The model under review builds one solid part; all positions refer to its coordinate system, in mm. Face numbers are marked on the shaded views. A direction names the side the tool comes from. Coordinates: 2 decimals unless noted, no trailing zeros. Loops run counter-clockwise (first coordinate to the right, second up) from the corner with the lowest first, then second, coordinate; pieces in that order, holes last. Notation, with made-up numbers: M 33.5,8.25 L 76.5,8.25 A24 ccw 76.5,38.25 Z; hole C 46,1.25 d6. An arc over 180 degrees is marked long. Return JSON: item names as keys, results as strings.
```python
from build123d import *

# Parameters (mm, degrees)
SKETCH1_R               = 9.35355
BOSS_EXTRUDE1_DEPTH     = 2.38125
BOSS_EXTRUDE2_START     = 6.35
SKETCH2_R               = 9.35355
SKETCH2_W               = 3.429
SKETCH2_H               = 3.429
BOSS_EXTRUDE2_DEPTH     = 6.35
SKETCH3_W               = 3.429
SKETCH3_H               = 3.429
SKETCH3_R               = 1.25
BOSS_EXTRUDE3_DEPTH     = 1
CUT_EXTRUDE1_DEPTH      = 20.29812849
CUT_EXTRUDE1_DEPTH_BACK = 20.29812849
SKETCH4_OUTSIDE_W       = 26.28
SKETCH4_OUTSIDE_H       = 26.279
SKETCH4_OUTSIDE_R       = 7.14375


with BuildPart() as part:
    # Sketch1 → Boss-Extrude1 (new body)
    with BuildSketch(Plane.XY.offset(20.11015)):
        with Locations((0, 5.0927)):
            Circle(SKETCH1_R)
        with BuildLine():
            Line((-2.032, 2.088352317), (-2.032, -1.4351))
            ThreePointArc((-2.032, -1.4351), (0, -3.4671), (2.032, -1.4351))
            Line((2.032, -1.4351), (2.032, 2.088352317))
            ThreePointArc((2.032, 2.088352317), (3.627, 5.0927), (2.032, 8.097047683))
            Line((2.032, 8.097047683), (2.032, 11.6205))
            ThreePointArc((2.032, 11.6205), (0, 13.6525), (-2.032, 11.6205))
            Line((-2.032, 11.6205), (-2.032, 8.097047683))
            ThreePointArc((-2.032, 8.097047683), (-3.627, 5.0927), (-2.032, 2.088352317))
        make_face(mode=Mode.SUBTRACT)
    extrude(amount=-BOSS_EXTRUDE1_DEPTH)

    # Sketch2 → Boss-Extrude2 (add)
    with BuildSketch(Plane.XY.offset(20.11015).offset(BOSS_EXTRUDE2_START)):
        with Locations((0, 5.0927)):
            Circle(SKETCH2_R)
        with Locations((0, 5.0927)):
            Rectangle(SKETCH2_W, SKETCH2_H, mode=Mode.SUBTRACT)
    extrude(amount=-BOSS_EXTRUDE2_DEPTH)

    # Sketch3 → Boss-Extrude3 (add)
    with BuildSketch(Plane(origin=(0, 0, 20.11015), x_dir=(-1, 0, 0), z_dir=(0, 0, -1))):
        with Locations((0, 5.0927)):
            Rectangle(SKETCH3_W, SKETCH3_H)
        with Locations((0, 5.0927)):
            Circle(SKETCH3_R, mode=Mode.SUBTRACT)
    extrude(amount=-BOSS_EXTRUDE3_DEPTH)

    # Sketch4 outside → Cut-Extrude1 (cut, two sides: drawn at the far end of the back side and taken through both)
    with BuildSketch(Plane(origin=(0, 0, 17.7289), x_dir=(-1, 0, 0), z_dir=(0, 0, -1)).offset(-CUT_EXTRUDE1_DEPTH_BACK)):
        with Locations((0, 5.0925)):
            Rectangle(SKETCH4_OUTSIDE_W, SKETCH4_OUTSIDE_H)
        with Locations((0, 5.0927)):
            Circle(SKETCH4_OUTSIDE_R, mode=Mode.SUBTRACT)
    extrude(amount=CUT_EXTRUDE1_DEPTH + CUT_EXTRUDE1_DEPTH_BACK, mode=Mode.SUBTRACT)


solid = part.part
```
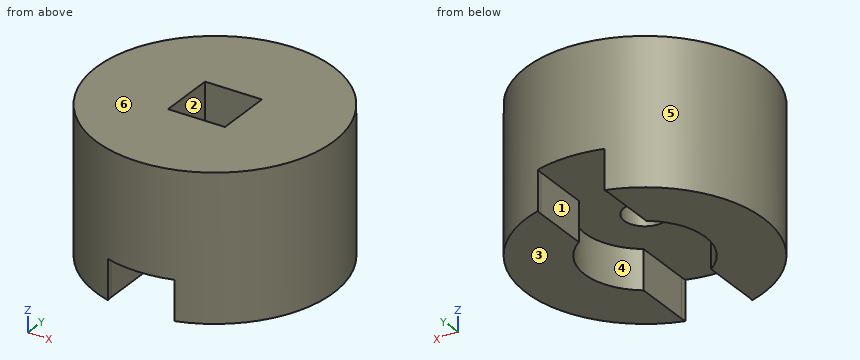
1. The part is to be moulded in two halves that separate along X. For the marked faces 4, 5 and 6, say which applies: released by +X, released by -X, zero draft, split by the parting line, or undercut.
Check values:
{"face 4": "undercut", "face 5": "split by the parting line", "face 6": "zero draft"}
2. Add section D-D on y = 0. Give the boundary of the cut face in (x, z), plus the area to 3 significant figures.
Check values:
{"outline": "M -5.01,17.73 L -2.03,17.73 L -2.03,20.11 L 2.03,20.11 L 2.03,17.73 L 5.01,17.73 L 5.01,26.46 L -5.01,26.46 Z", "area": "77.8 mm²"}
3. To check wall thickness, follow line 1 (Y direction, x = 0, z = 20.3); line 2 (X direction, y = 5, z = 21); line 3 (Z direction, x = -2.75, y = 3.25). State the ranges of each line that lie inside material, in increasing order.
Check values:
{"line 1": "-2.05 to 3.84, 6.34 to 12.24", "line 2": "-7.14 to -1.25, 1.25 to 7.14", "line 3": "20.11 to 26.46"}
4. Add section A-A on x = 0. Give the boundary of the cut face in (y, z), plus the area to 3 significant figures.
Check values:
{"outline": "M -2.05,20.11 L 3.84,20.11 L 3.84,21.11 L 3.38,21.11 L 3.38,26.46 L -2.05,26.46 Z; M 6.34,20.11 L 12.24,20.11 L 12.24,26.46 L 6.81,26.46 L 6.81,21.11 L 6.34,21.11 Z", "area": "69.9 mm²"}
5. Add section C-C on z = 25.5. Give the boundary of the cut face in (x, y).
Check values:
{"outline": "C 0,5.09 d14.29; hole M -1.71,3.38 L 1.71,3.38 L 1.71,6.81 L -1.71,6.81 Z"}
6. Machinability: for the marked faces 1, 2 and 3, which of the approach directions +Z, -Z, +X, -X, +Y, -Y give a long, thin tool a straight path to every point of the face, cutting with its end or side? Answer none if there is none.
Check values:
{"face 1": "-Z", "face 2": "+Z", "face 3": "-Z, +X, -X, +Y, -Y"}
7. Add section B-B on z = 18.5. Give the boundary of the cut face in (x, y).
Check values:
{"outline": "M -2.03,-1.44 L -2.03,2.09 A3.63 cw -2.03,8.1 L -2.03,11.62 A2.03 cw -2.01,11.95 A7.14 ccw -2.01,-1.76 A2.03 cw Z; M 2.01,-1.76 A7.14 ccw 2.01,11.95 A2.03 cw 2.03,11.62 L 2.03,8.1 A3.63 cw 2.03,2.09 L 2.03,-1.44 A2.03 cw Z"}
8. Insertion check: pin 1 Ø3 at (x, y) = (0, 5.09) entering from -Z; pin 2 Ø0.7 at (y, z) = (1, 19) entering from -X; pin 3 Ø2.5 at (y, z) = (9.5, 19.5) entering from +X. Each pin has a flat end and moves straight along its axis. Give the tip position at first contact, or say it passes through.
Check values:
{"pin 1": "z = 20.11", "pin 2": "x = -6.08", "pin 3": "x = 6.41"}
